```python
from build123d import *

# Parameters (mm, degrees)
SKETCH_1_R          = 10
EXTRUDE_1_DEPTH     = 2
SKETCH_2_R          = 1.5
CUT_EXTRUDE_1_DEPTH = 2
SKETCH_3_R          = 4.5
SKETCH_3_R_2        = 2.5
EXTRUDE_2_DEPTH     = 2.5


with BuildPart() as part:
    # 草图1 → 凸台-拉伸1 (new body)
    with BuildSketch(Plane(origin=(0, 0, 0), x_dir=(1, 0, 0), z_dir=(0, 1, 0))):
        Circle(SKETCH_1_R)
    extrude(amount=EXTRUDE_1_DEPTH)

    # 草图2 → 切除-拉伸1 (cut)
    with BuildSketch(Plane(origin=(0, 2, 0), x_dir=(1, 0, 0), z_dir=(0, 1, 0))):
        Circle(SKETCH_2_R)
        with Locations((0, 7)):
            Circle(SKETCH_2_R)
        with Locations((7, 0)):
            Circle(SKETCH_2_R)
        with Locations((0, -7)):
            Circle(SKETCH_2_R)
        with Locations((-7, 0)):
            Circle(SKETCH_2_R)
    extrude(amount=-CUT_EXTRUDE_1_DEPTH, mode=Mode.SUBTRACT)

    # 草图3 → 凸台-拉伸2 (add)
    with BuildSketch(Plane(origin=(0, 2, 0), x_dir=(1, 0, 0), z_dir=(0, 1, 0))):
        Circle(SKETCH_3_R)
        Circle(SKETCH_3_R_2, mode=Mode.SUBTRACT)
    extrude(amount=EXTRUDE_2_DEPTH)


solid = part.part
```
The model under review builds one solid part; all positions refer to its coordinate system, in mm. A direction names the side the tool comes from. Round coordinates to 2 decimals unless told otherwise and drop trailing zeros. Loops run counter-clockwise (first coordinate to the right, second up) from the corner with the lowest first, then second, coordinate; pieces in that order, holes last.
Item 1: For faces 1 (the face through (0, 2, 2)), 2 (the face through (-0.325, 1.014, 8.464)), list the 3-axis set-ups (+Z, -Z, +X, -X, +Y, -Y) from which the entire face can be reached by the end or side of a thin tool; tool diameter is ignored.
Determined:
face 1: +Y
face 2: +Y, -Y
Item 2: Take a section at D-D (y = 1.4). Write out the cut boundary in (x, z).
Determined:
outline: circle Ø20 at (0, 0); hole circle Ø3 at (-7, 0); hole circle Ø3 at (0, -7); hole circle Ø3 at (0, 0); hole circle Ø3 at (0, 7); hole circle Ø3 at (7, 0)
Item 3: For line 1 (Z direction, x = 0, y = 1.35); line 2 (X direction, y = 2.7, z = 0); line 3 (Y direction, x = -3.5, z = 3.5), list the stretches that pass through material, from the lowest coordinate up.
Determined:
line 1: z = -10 to -8.5, -5.5 to -1.5, 1.5 to 5.5, 8.5 to 10
line 2: x = -4.5 to -2.5, 2.5 to 4.5
line 3: y = 0 to 2
Item 4: Mouldability with a two-part tool opening along Z and no side actions: class faces 3 (the face through (-0.59, 3.23, -4.46)), 4 (the face through (4.3, 2, 2.1)), 5 (the face through (5.5, 1.01, -0.07)) as released by +Z, released by -Z, zero draft, split by the parting line, or undercut.
Determined:
face 3: split by the parting line
face 4: zero draft
face 5: undercut
Item 5: Take a section at A-A (z = 0). Write out the cut boundary in (x, y).
Determined:
outline: (-10, 0) - (-8.5, 0) - (-8.5, 2) - (-10, 2) - close; (-5.5, 0) - (-1.5, 0) - (-1.5, 2) - (-2.5, 2) - (-2.5, 4.5) - (-4.5, 4.5) - (-4.5, 2) - (-5.5, 2) - close; (1.5, 0) - (5.5, 0) - (5.5, 2) - (4.5, 2) - (4.5, 4.5) - (2.5, 4.5) - (2.5, 2) - (1.5, 2) - close; (8.5, 0) - (10, 0) - (10, 2) - (8.5, 2) - close
Item 6: Take a section at C-C (z = 6.5). Write out the cut boundary in (x, y).
Determined:
outline: (-7.6, 0) - (-1.41, 0) - (-1.41, 2) - (-7.6, 2) - close; (1.41, 0) - (7.6, 0) - (7.6, 2) - (1.41, 2) - close
Item 7: Take a section at B-B (x = 0.75). Write out the cut boundary in (y, z), then the cut area to 3 significant figures.
Determined:
outline: (0, -9.97) - (2, -9.97) - (2, -8.3) - (0, -8.3) - close; (0, -5.7) - (2, -5.7) - (2, -4.44) - (4.5, -4.44) - (4.5, -2.38) - (2, -2.38) - (2, -1.3) - (0, -1.3) - close; (0, 1.3) - (2, 1.3) - (2, 2.38) - (4.5, 2.38) - (4.5, 4.44) - (2, 4.44) - (2, 5.7) - (0, 5.7) - close; (0, 8.3) - (2, 8.3) - (2, 9.97) - (0, 9.97) - close
area: 34.6 mm2
Item 8: Clearance check with flat-ended pins moving along their axes: pin 1 Ø1.5 at (x, z) = (-1, 0) entering from +Y; pin 2 Ø2.5 at (x, z) = (7, 0) entering from -Y; pin 3 Ø1.5 at (y, z) = (1.5, -3.5) entering from -X. State where each tip first meets the part, or that it passes through.
Determined:
pin 1: stops at y = 2
pin 2: passes through
pin 3: stops at x = -9.61
